```python
from build123d import *

# Parameters (mm, degrees)
BOSS_EXTRUDE1_DEPTH      = 6
SKETCH3_R                = 19.1
CUT_EXTRUDE1_DEPTH       = 6
M5_CLEARANCE_HOLE1_D     = 5.3
CUT_EXTRUDE2_DEPTH       = 6
CUT_EXTRUDE4_DEPTH       = 6
F_5_0_5_DIAMETER_HOLE4_D = 5
M5_CLEARANCE_HOLE2_D     = 5.3
M5_CLEARANCE_HOLE2_DEPTH = 10
M5_CLEARANCE_HOLE2_TIP   = 1.59228064


with BuildPart() as part:
    # Sketch1 → Boss-Extrude1 (new body)
    with BuildSketch(Plane.XY):
        with BuildLine():
            Line((-55, -85), (55, -85))
            ThreePointArc((55, -85), (58.535533906, -83.535533906), (60, -80))
            Line((60, -80), (60, 80))
            ThreePointArc((60, 80), (58.535533906, 83.535533906), (55, 85))
            Line((55, 85), (-55, 85))
            ThreePointArc((-55, 85), (-58.535533906, 83.535533906), (-60, 80))
            Line((-60, 80), (-60, -80))
            ThreePointArc((-60, -80), (-58.535533906, -83.535533906), (-55, -85))
        make_face()
    extrude(amount=BOSS_EXTRUDE1_DEPTH)

    # Sketch3 → Cut-Extrude1 (cut)
    with BuildSketch(Plane.XY.offset(6)):
        with Locations((0, 45)):
            Circle(SKETCH3_R)
    extrude(amount=-CUT_EXTRUDE1_DEPTH, mode=Mode.SUBTRACT)

    # M5 Clearance Hole1 (through all)
    with Locations(Plane.XY.offset(6)):
        with Locations((-23.57, 68.57), (23.57, 68.57), (23.57, 21.43), (-23.57, 21.43)):
            Hole(M5_CLEARANCE_HOLE1_D / 2)

    # Sketch11 → Cut-Extrude2 (cut)
    with BuildSketch(Plane.XY.offset(6)):
        with BuildLine():
            Line((-43.03, 24.93), (-43.03, 17.93))
            ThreePointArc((-43.03, 17.93), (-45.57, 15.39), (-48.11, 17.93))
            Line((-48.11, 17.93), (-48.11, 24.93))
            ThreePointArc((-48.11, 24.93), (-45.57, 27.47), (-43.03, 24.93))
        make_face()
        with BuildLine():
            Line((43.03, 24.93), (43.03, 17.93))
            ThreePointArc((43.03, 17.93), (45.57, 15.39), (48.11, 17.93))
            Line((48.11, 17.93), (48.11, 24.93))
            ThreePointArc((48.11, 24.93), (45.57, 27.47), (43.03, 24.93))
        make_face()
    extrude(amount=-CUT_EXTRUDE2_DEPTH, mode=Mode.SUBTRACT)

    # Sketch15 → Cut-Extrude4 (cut)
    with BuildSketch(Plane.XY.offset(6)):
        with BuildLine():
            Line((-51.46, 47.54), (-46.46, 47.54))
            ThreePointArc((-46.46, 47.54), (-43.92, 45), (-46.46, 42.46))
            Line((-46.46, 42.46), (-51.46, 42.46))
            ThreePointArc((-51.46, 42.46), (-54, 45), (-51.46, 47.54))
        make_face()
        with BuildLine():
            Line((-51.46, 57.54), (-46.46, 57.54))
            ThreePointArc((-46.46, 57.54), (-43.92, 55), (-46.46, 52.46))
            Line((-46.46, 52.46), (-51.46, 52.46))
            ThreePointArc((-51.46, 52.46), (-54, 55), (-51.46, 57.54))
        make_face()
        with BuildLine():
            Line((51.46, 47.54), (46.46, 47.54))
            ThreePointArc((46.46, 47.54), (43.92, 45), (46.46, 42.46))
            Line((46.46, 42.46), (51.46, 42.46))
            ThreePointArc((51.46, 42.46), (54, 45), (51.46, 47.54))
        make_face()
        with BuildLine():
            Line((51.46, 57.54), (46.46, 57.54))
            ThreePointArc((46.46, 57.54), (43.92, 55), (46.46, 52.46))
            Line((46.46, 52.46), (51.46, 52.46))
            ThreePointArc((51.46, 52.46), (54, 55), (51.46, 57.54))
        make_face()
    extrude(amount=-CUT_EXTRUDE4_DEPTH, mode=Mode.SUBTRACT)

    # Ø5.0 (5) Diameter Hole4 (through all)
    with Locations(Plane.XY.offset(6)):
        with Locations((-45.57, -39.97), (45.57, -39.97), (20, -73), (0, -73), (-20, -73)):
            Hole(F_5_0_5_DIAMETER_HOLE4_D / 2)

    # M5 Clearance Hole2
    with Locations(Plane(origin=(0, 0, 0), x_dir=(-1, 0, 0), z_dir=(0, 0, -1))):
        with Locations((0, -53)):
            Hole(M5_CLEARANCE_HOLE2_D / 2, depth=M5_CLEARANCE_HOLE2_DEPTH)
            with Locations((0, 0, -(M5_CLEARANCE_HOLE2_DEPTH + M5_CLEARANCE_HOLE2_TIP / 2))):  # 118° drill point
                Cone(0, M5_CLEARANCE_HOLE2_D / 2, M5_CLEARANCE_HOLE2_TIP, mode=Mode.SUBTRACT)


solid = part.part
```
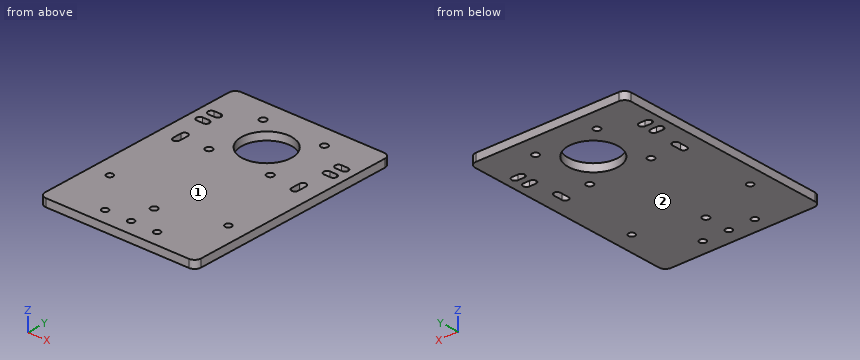
For this review, take the finished solid that the model builds, in its own axes (mm). Face numbers are marked on the shaded views. Coordinates: 2 decimals unless noted, no trailing zeros. Write each loop counter-clockwise with the first axis right and the second up, starting at its lowest first coordinate (ties: lowest second). Pieces come first, ordered by that corner, then holes. Notation, with made-up numbers: (61, 27.25) -> (90, 27.25) arc R21 cw to (90, 40.25) -> close; hole circle Ø5 at (78, 26.25). An arc over 180 degrees is marked (long way). Put each result on its own line as item: value.
Q1. Take a section at D-D, the plane z = 1.1. Count the separate pieces of the cut face and the enclosed holes in it, then the cut area to 3 significant figures.
From the geometry:
separate pieces: 1
enclosed holes: 17
area: 18,700 mm2
Q2. Clearance check with a flat-ended pin moving along its axis: pin 1 Ø3 at (x, y) = (0, -53) entering from +Z (1 decimal). State where the tip first meets the part, or that it passes through.
From the geometry:
pin 1: passes through
Q3. Take a section at C-C, the plane x = 13. State the section outline as (y, z) points, then the cut area to 3 significant figures.
From the geometry:
outline: (-85, 0) -> (31.01, 0) -> (31.01, 6) -> (-85, 6) -> close; (58.99, 0) -> (85, 0) -> (85, 6) -> (58.99, 6) -> close
area: 852 mm2
Q4. The part is to be moulded in two halves that separate along Z. For the marked faces 1 and 2, say which applies: +Z half, -Z half, draft (parallel to the pull), parting line (faces both ways), or undercut.
From the geometry:
face 1: +Z half
face 2: -Z half
Q5. Wall thickness on L1, parallel to X at y = 18.5, z = 1.5; L2, parallel to Y at x = 51.5, z = 4.8; L3, parallel to Y at x = -23.57, z = 3.15: over which ranges is each line inside the solid? List them lowest first.
From the geometry:
L1: x = -60 to -48.11, -43.03 to 43.03, 48.11 to 60
L2: y = -85 to 42.46, 47.54 to 52.46, 57.54 to 85
L3: y = -85 to 18.78, 24.08 to 65.92, 71.22 to 85
Q6. Take a section at A-A, the plane y = 21.43. State the section outline as (x, z) points, then the cut area to 3 significant figures.
From the geometry:
outline: (-60, 0) -> (-48.11, 0) -> (-48.11, 6) -> (-60, 6) -> close; (-43.03, 0) -> (-26.22, 0) -> (-26.22, 6) -> (-43.03, 6) -> close; (-20.92, 0) -> (20.92, 0) -> (20.92, 6) -> (-20.92, 6) -> close; (26.22, 0) -> (43.03, 0) -> (43.03, 6) -> (26.22, 6) -> close; (48.11, 0) -> (60, 0) -> (60, 6) -> (48.11, 6) -> close
area: 595 mm2
Q7. Take a section at B-B, the plane y = 68.57. State the section outline as (x, z) points.
From the geometry:
outline: (-60, 0) -> (-26.22, 0) -> (-26.22, 6) -> (-60, 6) -> close; (-20.92, 0) -> (20.92, 0) -> (20.92, 6) -> (-20.92, 6) -> close; (26.22, 0) -> (60, 0) -> (60, 6) -> (26.22, 6) -> close
